Source: CAD feature listing. Evaluate the final solid. Frame: model axes, mm. A direction names the side the tool comes from. Give positions to 0.01 mm unless a question says otherwise; leave off trailing zeros. Order: outer loops, then holes, each group sorted by start corner. A loop starts at its lowest first (then second) coordinate and runs counter-clockwise, first axis right, second up. Notation, with made-up numbers: M -12.5,0.25 L 18.5,0.25 A9 ccw 18.5,10.25 Z; hole C 75,89.25 d3. An arc over 180 degrees is marked long. Use CSV: the item, a comma, the result in double quotes. Start each with the question number.
Item 1: First-contact query: pin 1 (1.6 mm diameter, centred on y = 1.5, z = -87.5, fed in from -X); pin 2 (1.5 mm diameter, centred on x = 104, y = 2.5, fed in from -Z); pin 3 (1.5 mm diameter, centred on x = 95.5, y = 1.5, fed in from +Z). Flat tips, straight axial feed; report the tip coordinate or a pass-through.
Item 2: Ray query, probe 1 along Z at (x, y) = (19.05, 0.8); probe 2 along Z at (x, y) = (53, 0.25); probe 3 along Z at (x, y) = (31.75, 2.55). Return the intervals inside material, ascending. Write a range as from..to.
Item 3: Section query D-D on x = 19.05. Return loops of the section in (y, z) (3 decimals), and give its area (3 significant figures).
Item 4: Section query B-B on y = 1.85. Count the separate pieces of the cut face and the enclosed holes in it, and give its area (3 significant figures).
Item 5: Section query C-C on z = -40. Return loops of the section in (x, y) (3 decimals), and give its area (3 significant figures).
Item 6: Section query A-A on x = 44.45. Return loops of the section in (y, z) (3 decimals).
Item 7: Access query for faces 1 (the face through (32, 2, -95.25)), 2 (the face through (92, 2, -165.1)), 3 (the face through (122.432, 1.565, 0.332)), 4 (the face through (121.932, 2, -136)), 5 (the face through (0, 2, -34)). Directions: +Z, -Z, +X, -X, +Y, -Y. A direction counts if a zero-diameter tool reaches every point of the face in a straight line with its end or side. Return the directions, or none.
from build123d import *

# Parameters (mm, degrees)
SKETCH1_R           = 2.2479
BOSS_EXTRUDE1_DEPTH = 3.175
SKETCH2_R           = 2.4892
SKETCH2_R_2         = 2.2479
CUT_EXTRUDE1_DEPTH  = 4.175
SKETCH3_R           = 1.778
CUT_EXTRUDE2_DEPTH  = 4.175


with BuildPart() as part:
    # Sketch1 → Boss-Extrude1 (new body)
    with BuildSketch(Plane(origin=(0, 0, 0), x_dir=(1, 0, 0), z_dir=(0, 1, 0))):
        with BuildLine():
            Line((0, 165.1), (61.874509804, 165.1))
            ThreePointArc((61.874509804, 165.1), (65.840083533, 167.005), (69.805657262, 165.1))
            Line((69.805657262, 165.1), (114.791176471, 165.1))
            ThreePointArc((114.791176471, 165.1), (122.348852648, 165.517102448), (121.9317502, 157.959426271))
            Line((121.9317502, 157.959426271), (121.9317502, 112.973907062))
            ThreePointArc((121.9317502, 112.973907062), (123.8367502, 109.008333333), (121.9317502, 105.042759604))
            Line((121.9317502, 105.042759604), (121.9317502, 60.057240396))
            ThreePointArc((121.9317502, 60.057240396), (123.8367502, 56.091666667), (121.9317502, 52.126092938))
            Line((121.9317502, 52.126092938), (121.9317502, 7.140573729))
            ThreePointArc((121.9317502, 7.140573729), (122.348852648, -0.417102448), (114.791176471, 0))
            Line((114.791176471, 0), (69.805657262, 0))
            ThreePointArc((69.805657262, 0), (65.840083533, -1.905), (61.874509804, 0))
            Line((61.874509804, 0), (0, 0))
            Line((0, 0), (0, 69.85))
            Line((0, 69.85), (63.5, 69.72449217))
            Line((63.5, 69.72449217), (63.5, 95.25))
            Line((63.5, 95.25), (0, 95.25))
            Line((0, 95.25), (0, 165.1))
        make_face()
        with Locations((65.840083533, 3.175)):
            Circle(SKETCH1_R, mode=Mode.SUBTRACT)
        with Locations((118.7567502, 3.175)):
            Circle(SKETCH1_R, mode=Mode.SUBTRACT)
        with Locations((118.7567502, 56.091666667)):
            Circle(SKETCH1_R, mode=Mode.SUBTRACT)
        with Locations((118.7567502, 109.008333333)):
            Circle(SKETCH1_R, mode=Mode.SUBTRACT)
        with Locations((118.7567502, 161.925)):
            Circle(SKETCH1_R, mode=Mode.SUBTRACT)
        with Locations((65.840083533, 161.925)):
            Circle(SKETCH1_R, mode=Mode.SUBTRACT)
    extrude(amount=BOSS_EXTRUDE1_DEPTH)

    # Sketch2 → Cut-Extrude1 (cut, through all)
    with BuildSketch(Plane.XZ):
        with Locations((19.05, -50.762310441)):
            Circle(SKETCH2_R)
        with Locations((19.05, -114.3)):
            Circle(SKETCH2_R)
        with Locations((31.75, -65.024736783)):
            Circle(SKETCH2_R_2)
        with Locations((96.5317502, -64.896695572)):
            Circle(SKETCH2_R_2)
        with Locations((96.493890617, -100.14870612)):
            Circle(SKETCH2_R_2)
        with Locations((31.712564881, -99.881518123)):
            Circle(SKETCH2_R_2)
    extrude(amount=-CUT_EXTRUDE1_DEPTH, mode=Mode.SUBTRACT)

    # Sketch3 → Cut-Extrude2 (cut, through all)
    with BuildSketch(Plane(origin=(0, 3.175, 0), x_dir=(1, 0, 0), z_dir=(0, 1, 0))):
        with Locations((44.45, 9.525)):
            Circle(SKETCH3_R)
        with Locations((44.45, 50.525)):
            Circle(SKETCH3_R)
    extrude(amount=-CUT_EXTRUDE2_DEPTH, mode=Mode.SUBTRACT)


solid = part.part
Verdict:
1,pin 1,"x = 63.5"
1,pin 2,"z = -165.1"
1,pin 3,"z = 0"
2,probe 1,"-165.1..-116.79, -111.81..-95.25, -69.81..-53.25, -48.27..0"
2,probe 2,"-165.1..-95.25, -69.75..0"
2,probe 3,"-165.1..-102.13, -97.63..-95.25, -69.79..-67.27, -62.78..0"
3,outline,"M 0,-165.1 L 3.175,-165.1 L 3.175,-116.789 L 0,-116.789 Z; M 0,-111.811 L 3.175,-111.811 L 3.175,-95.25 L 0,-95.25 Z; M 0,-69.812 L 3.175,-69.812 L 3.175,-53.252 L 0,-53.252 Z; M 0,-48.273 L 3.175,-48.273 L 3.175,0 L 0,0 Z"
3,area,"412 mm2"
4,separate pieces,"1"
4,enclosed holes,"14"
4,area,"18,400 mm2"
5,outline,"M 0,0 L 121.932,0 L 121.932,3.175 L 0,3.175 Z"
5,area,"387 mm2"
6,outline,"M 0,-165.1 L 3.175,-165.1 L 3.175,-95.25 L 0,-95.25 Z; M 0,-69.762 L 3.175,-69.762 L 3.175,-52.303 L 0,-52.303 Z; M 0,-48.747 L 3.175,-48.747 L 3.175,-11.303 L 0,-11.303 Z; M 0,-7.747 L 3.175,-7.747 L 3.175,0 L 0,0 Z"
7,face 1,"-X, +Y, -Y"
7,face 2,"-Z, +Y, -Y"
7,face 3,"+Y, -Y"
7,face 4,"+X, +Y, -Y"
7,face 5,"+Z, -Z, -X, +Y, -Y"
